from build123d import *

# Parameters (mm, degrees)
SKETCH1_W           = 70.75
SKETCH1_H           = 54.34
PCB_DEPTH           = 1.6
SKETCH2_W           = 69.15
SKETCH2_H           = 50
SCREEN_DEPTH        = 3.7
SKETCH3_W           = 59.5
SKETCH3_H           = 45.5
USABLE_SPACE_DEPTH  = 0.01
SKETCH4_W           = 16.823482751
SKETCH4_H           = 14.30589821
SD_SLOT_DEPTH       = 2.8
SKETCH6_W           = 6.52491574
SKETCH6_H           = 6.37715793
RESET_BUTTON_DEPTH  = 2.19
BOSS_EXTRUDE6_DEPTH = 1.23
SKETCH8_W           = 5.544724278
SKETCH8_H           = 7.737048543
BOSS_EXTRUDE7_DEPTH = 7.75
SKETCH9_W           = 20.155505067
SKETCH9_H           = 2.546724467
SKETCH9_W_2         = 15.280346801
SKETCH9_W_3         = 25.321717556
SKETCH9_H_2         = 2.837778691
SKETCH9_W_4         = 20.737613516
PINS_DEPTH          = 2.15


with BuildPart() as part:
    # Sketch1 → PCB (new body)
    with BuildSketch(Plane(origin=(0, 0, 0), x_dir=(1, 0, 0), z_dir=(0, 1, 0))):
        with Locations((35.375, 27.17)):
            Rectangle(SKETCH1_W, SKETCH1_H)
    extrude(amount=PCB_DEPTH)

    # Sketch2 → Screen (add)
    with BuildSketch(Plane(origin=(0, 1.6, 0), x_dir=(1, 0, 0), z_dir=(0, 1, 0))):
        with Locations((34.575, 27.6)):
            Rectangle(SKETCH2_W, SKETCH2_H)
    extrude(amount=SCREEN_DEPTH)

    # Sketch3 → usable space (add)
    with BuildSketch(Plane(origin=(0, 5.3, 0), x_dir=(1, 0, 0), z_dir=(0, 1, 0))):
        with Locations((32.25, 28.25)):
            Rectangle(SKETCH3_W, SKETCH3_H)
    extrude(amount=USABLE_SPACE_DEPTH)

    # Sketch4 → SD slot (add)
    with BuildSketch(Plane.XZ):
        with Locations((8.411741376, -22.818507851)):
            Rectangle(SKETCH4_W, SKETCH4_H)
    extrude(amount=SD_SLOT_DEPTH)

    # Sketch6 → reset button (add)
    with BuildSketch(Plane.XZ):
        with Locations((5.542908416, -51.151421035)):
            Rectangle(SKETCH6_W, SKETCH6_H)
    extrude(amount=RESET_BUTTON_DEPTH)

    # Sketch7 → Boss-Extrude6 (add)
    with BuildSketch(Plane.XZ.offset(2.19)):
        with BuildLine():
            ThreePointArc((5.542908416, -49.571421035), (4.425679702, -50.034192321), (3.962908416, -51.151421035))
            Line((3.962908416, -51.151421035), (5.542908416, -51.151421035))
            Line((5.542908416, -51.151421035), (5.542908416, -49.571421035))
        make_face()
        with BuildLine():
            Line((5.542908416, -51.151421035), (3.962908416, -51.151421035))
            ThreePointArc((3.962908416, -51.151421035), (4.425679702, -52.268649749), (5.542908416, -52.731421035))
            Line((5.542908416, -52.731421035), (5.542908416, -51.151421035))
        make_face()
        with BuildLine():
            Line((5.542908416, -49.571421035), (5.542908416, -51.151421035))
            Line((5.542908416, -51.151421035), (7.122908416, -51.151421035))
            ThreePointArc((7.122908416, -51.151421035), (6.66013713, -50.034192321), (5.542908416, -49.571421035))
        make_face()
        with BuildLine():
            Line((7.122908416, -51.151421035), (5.542908416, -51.151421035))
            Line((5.542908416, -51.151421035), (5.542908416, -52.731421035))
            ThreePointArc((5.542908416, -52.731421035), (6.66013713, -52.268649749), (7.122908416, -51.151421035))
        make_face()
    extrude(amount=BOSS_EXTRUDE6_DEPTH)

    # Sketch8 → Boss-Extrude7 (add)
    with BuildSketch(Plane.XZ):
        with Locations((65.962973945, -28.471475729)):
            Rectangle(SKETCH8_W, SKETCH8_H)
    extrude(amount=BOSS_EXTRUDE7_DEPTH)

    # Sketch9 → pins (add)
    with BuildSketch(Plane.XZ):
        with Locations((37.084943571, -3.012499342)):
            Rectangle(SKETCH9_W, SKETCH9_H)
        with Locations((57.640648197, -3.012499342)):
            Rectangle(SKETCH9_W_2, SKETCH9_H)
        with Locations((30.572605291, -51.764081995)):
            Rectangle(SKETCH9_W_3, SKETCH9_H_2)
        with Locations((55.421359732, -51.764081995)):
            Rectangle(SKETCH9_W_4, SKETCH9_H_2)
    extrude(amount=PINS_DEPTH)


solid = part.part
Geometry: final body of the model. Coordinates: model frame, mm. A direction names the side the tool comes from. Round coordinates to 2 decimals unless told otherwise and drop trailing zeros. Order: outer loops, then holes, each group sorted by start corner. A loop starts at its lowest first (then second) coordinate and runs counter-clockwise, first axis right, second up. Notation, with made-up numbers: (-27.75, 72) -> (21.25, 72) arc R35 ccw to (21.25, 105) -> close; hole circle Ø1 at (50, 68). An arc over 180 degrees is marked (long way). Put each result on its own line as item: value. Start each with the question number.
Q1. Section A-A on y = -0.75. Return the cut outline in (x, z), and give its area (3 significant figures).
Q2. First-contact query: pin 1 (2.5 mm diameter, centred on y = -1.5, z = -51.5, fed in from -X); pin 2 (2 mm diameter, centred on y = -1.5, z = -24, fed in from +X); pin 3 (3 mm diameter, centred on y = -5.5, z = -32.5, fed in from -X). Flat tips, straight axial feed; report the tip coordinate or a pass-through.
Q3. Reachability of faces 1 (the flat face through (8.805, -1, -51)), 2 (the flat face through (30, -2.15, -52)), 3 (the flat face through (8, -1, -29.971)), 4 (the flat face through (37, -1, -1.739)), 5 (the flat face through (2.28, -1, -51)) from +Z, -Z, +X, -X, +Y, -Y: full face, straight path, thin tool, end or side. Return the list, or none.
Q4. Line query: probe 1 along X at (y, z) = (-0.5, -50.5); probe 2 along Z at (x, y) = (59.5, -1.75); probe 3 along Y at (x, z) = (60, -36.5). Output: solid intervals per line, ascending.
Q5. Section D-D on y = 3.5. Return the cut outline in (x, z), and give its area (3 significant figures).
Ans:
1. outline: (0, -29.97) -> (16.82, -29.97) -> (16.82, -15.67) -> (0, -15.67) -> close; (2.28, -54.34) -> (8.81, -54.34) -> (8.81, -47.96) -> (2.28, -47.96) -> close; (17.91, -53.18) -> (43.23, -53.18) -> (43.23, -50.35) -> (17.91, -50.35) -> close; (27.01, -4.29) -> (47.16, -4.29) -> (47.16, -1.74) -> (27.01, -1.74) -> close; (45.05, -53.18) -> (65.79, -53.18) -> (65.79, -50.35) -> (45.05, -50.35) -> close; (50, -4.29) -> (65.28, -4.29) -> (65.28, -1.74) -> (50, -1.74) -> close; (63.19, -32.34) -> (68.74, -32.34) -> (68.74, -24.6) -> (63.19, -24.6) -> close
1. area: 546 mm2
2. pin 1: stops at x = 2.28
2. pin 2: stops at x = 68.74
2. pin 3: stops at x = 63.19
3. face 1: -Z, -Y
3. face 2: +Z, -Z, +X, -Y
3. face 3: -X, -Y
3. face 4: +Z, +X, -X, -Y
3. face 5: -Z, -X, -Y
4. probe 1: x = 2.28 to 8.81, 17.91 to 43.23, 45.05 to 65.79
4. probe 2: z = -53.18 to -50.35, -4.29 to -1.74
4. probe 3: y = 0 to 5.31
5. outline: (0, -52.6) -> (69.15, -52.6) -> (69.15, -2.6) -> (0, -2.6) -> close
5. area: 3,460 mm2
